For this review, take the finished solid that the model builds, in its own axes (mm). Give positions to 0.01 mm unless a question says otherwise; leave off trailing zeros. Order: outer loops, then holes, each group sorted by start corner. A loop starts at its lowest first (then second) coordinate and runs counter-clockwise, first axis right, second up. Notation, with made-up numbers: M -3.75,59 L 21.25,59 A25 ccw 21.25,78 Z; hole C -18,13.25 d6. An arc over 180 degrees is marked long. Use CSV: the item, a comma, the result in double quotes. Start each with the question number.
(1) Clearance check with flat-ended pins moving along their axes: P1, Ø0.9, axis at x = 1, z = -2, coming from the -Y side; P2, Ø1.6, axis at x = 2, y = 11.5, coming from the -Z side; P3, Ø1.5, axis at x = 2, y = 11, coming from the +Z side. State where each tip first meets the part, or that it passes through.
(2) Wall thickness on L1, parallel to Y at x = 1.6, z = -2.5; L2, parallel to Y at x = 2.2, z = 18; L3, parallel to Y at x = 1.1, z = -21: over which ranges is each line inside the solid? List them lowest first. Write a range as from..to.
(3) Consider section B-B (y = 0). Write out the cut boundary in (x, z), and give its area (3 significant figures).
(4) Consider section C-C (z = -1.5). Write out the cut boundary in (x, y).
(5) Consider section D-D (x = 1.2). Give the number of separate pieces and of enclosed holes in the cut face, and give its area (3 significant figures).
(6) Consider section A-A (z = -21). Write out the cut boundary in (x, y), and give its area (3 significant figures).
```python
from build123d import *
from OCP.BRepFilletAPI import BRepFilletAPI_MakeFillet

# Parameters (mm, degrees)
SKETCH_1_R          = 1.55
EXTRUDE_1_DEPTH     = 3
FILLET_1_R1         = 1
FILLET_1_R2         = 2
SKETCH_2_W          = 23.55236831
SKETCH_2_H          = 10
CUT_EXTRUDE_1_DEPTH = 10


with BuildPart() as part:
    # Sketch 1 → Extrude 1 (new body)
    with BuildSketch(Plane(origin=(0, 0, 0), x_dir=(0, 0, -1), z_dir=(1, 0, 0))):
        with BuildLine():
            Line((-7, -10), (25, -10))
            Line((25, -10), (25, 10))
            Line((25, 10), (-7, 10))
            Line((-7, 10), (-7, 12.483339502))
            Line((-7, 12.483339502), (-20, 35))
            Line((-20, 35), (-25, 35))
            Line((-25, 35), (-25, 32.1))
            ThreePointArc((-25, 32.1), (-23.95, 31.05), (-25, 30))
            Line((-25, 30), (-28, 30))
            Line((-28, 30), (-28, 20))
            Line((-28, 20), (-25, 20))
            ThreePointArc((-25, 20), (-23.95, 18.95), (-25, 17.9))
            Line((-25, 17.9), (-25, 7.1))
            ThreePointArc((-25, 7.1), (-23.95, 6.05), (-25, 5))
            Line((-25, 5), (-28, 5))
            Line((-28, 5), (-28, -5))
            Line((-28, -5), (-25, -5))
            ThreePointArc((-25, -5), (-23.95, -6.05), (-25, -7.1))
            Line((-25, -7.1), (-25, -17.9))
            ThreePointArc((-25, -17.9), (-23.95, -18.95), (-25, -20))
            Line((-25, -20), (-28, -20))
            Line((-28, -20), (-28, -30))
            Line((-28, -30), (-25, -30))
            ThreePointArc((-25, -30), (-23.95, -31.05), (-25, -32.1))
            Line((-25, -32.1), (-25, -35))
            Line((-25, -35), (-20, -35))
            Line((-20, -35), (-7, -12.483339502))
            Line((-7, -12.483339502), (-7, -10))
        make_face()
        Polygon((-10.185045424, 10), (-20, 10), (-20, 27), align=None, mode=Mode.SUBTRACT)
        Polygon((-20, -10), (-10.185045424, -10), (-20, -27), align=None, mode=Mode.SUBTRACT)
        Polygon((12.493060906, -6), (-12.493060906, -6), (0, -1.590684386), align=None, mode=Mode.SUBTRACT)
        with Locations((-21, 0)):
            Circle(SKETCH_1_R, mode=Mode.SUBTRACT)
        Polygon((-4.506939094, 0), (-17, -4.409315614), (-17, 4.409315614), align=None, mode=Mode.SUBTRACT)
        Polygon((0, 1.590684386), (-12.493060906, 6), (12.493060906, 6), align=None, mode=Mode.SUBTRACT)
        Polygon((17, 4.409315614), (17, -4.409315614), (4.506939094, 0), align=None, mode=Mode.SUBTRACT)
        with Locations((21, 0)):
            Circle(SKETCH_1_R, mode=Mode.SUBTRACT)
    extrude(amount=EXTRUDE_1_DEPTH)

    # Fillet 1: one fillet with a radius per group of edges: ONE call of the kernel's fillet builder (fillet() takes one radius for all edges)
    fillet_1_edges_1 = [part.edges().sort_by_distance(p)[0] for p in [
        (1.5, -10, 10.185045424),
        (1.5, -10, 20),
        (1.5, 10, 10.185045424),
        (1.5, 10, 20),
        (1.5, 27, 20),
        (1.5, 10, 7),
        (1.5, 10, -25),
        (1.5, -10, -25),
        (1.5, -10, 7),
        (1.5, -4.409315614, 17),
        (1.5, 1.590684386, 0),
        (1.5, 6, 12.493060906),
        (1.5, 6, -12.493060906),
        (1.5, 4.409315614, 17),
        (1.5, 0, 4.506939094),
        (1.5, 0, -4.506939094),
        (1.5, 4.409315614, -17),
        (1.5, -4.409315614, -17),
        (1.5, -1.590684386, 0),
        (1.5, -6, -12.493060906),
        (1.5, -6, 12.493060906),
    ]]
    fillet_1_edges_2 = [part.edges().sort_by_distance(p)[0] for p in [
        (1.5, -27, 20),
    ]]
    fillet_1 = BRepFilletAPI_MakeFillet(part.part.solid().wrapped)
    for e in fillet_1_edges_1:
        fillet_1.Add(FILLET_1_R1, e.wrapped)
    for e in fillet_1_edges_2:
        fillet_1.Add(FILLET_1_R2, e.wrapped)
    add(Compound.cast(fillet_1.Shape()), mode=Mode.REPLACE)

    # Sketch 2 → Cut-Extrude 1 (cut)
    with BuildSketch(Plane(origin=(3, 0, 0), x_dir=(0, 0, -1), z_dir=(1, 0, 0))):
        with Locations((-22.372535414, -30)):
            Rectangle(SKETCH_2_W, SKETCH_2_H)
    extrude(amount=-CUT_EXTRUDE_1_DEPTH, mode=Mode.SUBTRACT)


solid = part.part
```
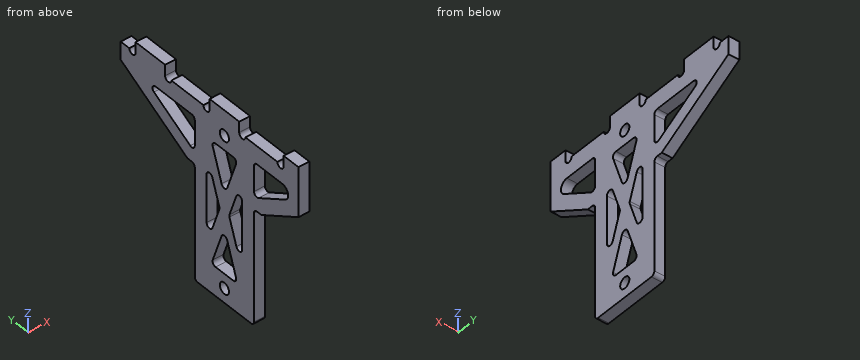
Check result:
1,P1,"stops at y = -10"
1,P2,"stops at z = 6.95"
1,P3,"stops at z = 25"
2,L1,"y = -10..-6, -2.47..2.47, 6..10"
2,L2,"y = -25..-21.54, -10..10, 23.54..31.54"
2,L3,"y = -10..-1.55, 1.55..10"
3,outline,"M 0,-25 L 3,-25 L 3,-22.55 L 0,-22.55 Z; M 0,-19.45 L 3,-19.45 L 3,-17 L 0,-17 Z; M 0,-6.51 L 3,-6.51 L 3,6.51 L 0,6.51 Z; M 0,17 L 3,17 L 3,19.45 L 0,19.45 Z; M 0,22.55 L 3,22.55 L 3,28 L 0,28 Z"
3,area,"77.5 mm^2"
4,outline,"M 0,-10 L 3,-10 L 3,-6 L 0,-6 Z; M 0,-2.12 L 3,-2.12 L 3,2.12 L 0,2.12 Z; M 0,6 L 3,6 L 3,10 L 0,10 Z"
5,separate pieces,"1"
5,enclosed holes,"8"
5,area,"1,230 mm^2"
6,outline,"M 0,-10 L 3,-10 L 3,-1.55 L 0,-1.55 Z; M 0,1.55 L 3,1.55 L 3,10 L 0,10 Z"
6,area,"50.7 mm^2"
